```python
from build123d import *

# Parameters (mm, degrees)
F2_W = 80.009996891
F2_H = 70.8002150059
F4_T = 2.54


# Not quite as in the source:
# - the arcs of a loft's sections are written as splines that run evenly, so that the points pair up as in the source's solid
# - a shell that OpenCascade refuses in one call is made with other operations: the cavity is built on its own and cut out


with BuildPart() as f3:
    # F2 (on offset) → F3 section 0
    with BuildSketch(Plane.XY.offset(127)):
        Rectangle(F2_W, F2_H)
    # F0 (on Top) → F3 section 1
    with BuildSketch(Plane.XY):
        with BuildLine():
            add(Edge.make_bspline(
                [(26.065590987, 23.0652358186), (24.5559748328, 24.7712247593), (22.8783749167, 26.3284909791), (19.2515124469, 29.085885659), (17.3023395745, 30.2859459372), (13.2072252341, 32.2827922844), (11.0613850258, 33.0795289775), (6.6553917622, 34.2390893068), (4.3953476538, 34.6018842705), (-0.1522046827, 34.8795973285), (-2.4396004636, 34.7945085558), (-6.953951987, 34.1797019856), (-9.1807961033, 33.6499993904), (-13.4884628163, 32.1662998637), (-15.5691788974, 31.2123396195), (-19.5046195839, 28.916764877), (-21.3592468778, 27.5752071412), (-23.0652358186, 26.065590987)],
                knots=[0, 0, 0, 0, 0.125, 0.125, 0.25, 0.25, 0.375, 0.375, 0.5, 0.5, 0.625, 0.625, 0.75, 0.75, 0.875, 0.875, 1, 1, 1, 1], degree=3))
            add(Edge.make_bspline(
                [(-23.0652358186, 26.065590987), (-24.7712247593, 24.5559748328), (-26.3284909791, 22.8783749167), (-29.085885659, 19.2515124469), (-30.2859459372, 17.3023395745), (-32.2827922844, 13.2072252341), (-33.0795289775, 11.0613850258), (-34.2390893068, 6.6553917622), (-34.6018842705, 4.3953476538), (-34.8795973285, -0.1522046827), (-34.7945085558, -2.4396004636), (-34.1797019856, -6.953951987), (-33.6499993904, -9.1807961033), (-32.1662998637, -13.4884628163), (-31.2123396195, -15.5691788974), (-28.916764877, -19.5046195839), (-27.5752071412, -21.3592468778), (-26.065590987, -23.0652358186)],
                knots=[0, 0, 0, 0, 0.125, 0.125, 0.25, 0.25, 0.375, 0.375, 0.5, 0.5, 0.625, 0.625, 0.75, 0.75, 0.875, 0.875, 1, 1, 1, 1], degree=3))
            add(Edge.make_bspline(
                [(-26.065590987, -23.0652358186), (-24.5559748328, -24.7712247593), (-22.8783749167, -26.3284909791), (-19.2515124469, -29.085885659), (-17.3023395745, -30.2859459372), (-13.2072252341, -32.2827922844), (-11.0613850258, -33.0795289775), (-6.6553917622, -34.2390893068), (-4.3953476538, -34.6018842705), (0.1522046827, -34.8795973285), (2.4396004636, -34.7945085558), (6.953951987, -34.1797019856), (9.1807961033, -33.6499993904), (13.4884628163, -32.1662998637), (15.5691788974, -31.2123396195), (19.5046195839, -28.916764877), (21.3592468778, -27.5752071412), (23.0652358186, -26.065590987)],
                knots=[0, 0, 0, 0, 0.125, 0.125, 0.25, 0.25, 0.375, 0.375, 0.5, 0.5, 0.625, 0.625, 0.75, 0.75, 0.875, 0.875, 1, 1, 1, 1], degree=3))
            add(Edge.make_bspline(
                [(23.0652358186, -26.065590987), (24.7712247593, -24.5559748328), (26.3284909791, -22.8783749167), (29.085885659, -19.2515124469), (30.2859459372, -17.3023395745), (32.2827922844, -13.2072252341), (33.0795289775, -11.0613850258), (34.2390893068, -6.6553917622), (34.6018842705, -4.3953476538), (34.8795973285, 0.1522046827), (34.7945085558, 2.4396004636), (34.1797019856, 6.953951987), (33.6499993904, 9.1807961033), (32.1662998637, 13.4884628163), (31.2123396195, 15.5691788974), (28.916764877, 19.5046195839), (27.5752071412, 21.3592468778), (26.065590987, 23.0652358186)],
                knots=[0, 0, 0, 0, 0.125, 0.125, 0.25, 0.25, 0.375, 0.375, 0.5, 0.5, 0.625, 0.625, 0.75, 0.75, 0.875, 0.875, 1, 1, 1, 1], degree=3))
        make_face()
    loft(ruled=True)

    # F4: shell of thickness 2.54, made by hand


with BuildPart() as f4_core1:
    # F4_t2: copy of F3
    add(f3.part)

    # the walls: a layer under each face that stays
    f4_faces = [f4_core1.faces().sort_by_distance(p)[0] for p in [
        (37.3728696225, -1.0607857428, 63.5),
        (1.0607857428, 35.0704241512, 63.5),
        (-37.3728696225, 1.0607857428, 63.5),
        (-1.0607857428, -35.0704241512, 63.5),
        (0, 0, 0),
    ]]
    thicken(f4_faces, amount=-F4_T, mode=Mode.SUBTRACT)


with BuildPart() as f3_1:
    add(f3.part)

    # what is left inside the walls is the cavity
    f4_cavity = [f4_core1.part.solids().sort_by_distance(p)[0] for p in [
        (-0.656082, -32.618968, 85.395704),
    ]]
    add(f4_cavity, mode=Mode.SUBTRACT)


solid = f3_1.part
```
Here's how the part is built. I have some questions about the finished solid (model axes, mm). Give positions to 0.01 mm unless a question says otherwise; leave off trailing zeros. Answer as a JSON object with one key per item and string values. Group by question number.
Item 1: If we mould it in two halves opening along X, with no side actions, what happens to faces 1 (the flat face through (-1, 0, 2.54)), 2 (the flat face through (-1, 0, 0))? For each: pulls with the +X half, pulls with the -X half, needs draft (parallel to the pull), parting line crosses it, or undercut.
Item 2: For P1, Ø4, axis at x = -30.5, z = 46.5, coming from the -Y side; P2, Ø4, axis at y = 14, z = 108.5, coming from the +X side; P3, Ø1, axis at x = 3.5, y = 0.5, coming from the +Z side, each with a flat end and sliding along its axis, tell me the tip position at first contact or that it passes through.
Item 3: Please list where these lines run through material, in increasing order: probe 1 along Z at (x, y) = (-26, 10.5); probe 2 along Y at (x, z) = (21, 66.5); probe 3 along X at (y, z) = (21, 116.5).
Result set:
{
 "1": {"face 1": "undercut", "face 2": "needs draft"},
 "2": {"P1": "y = -28.87", "P2": "x = 39.18", "P3": "z = 2.54"},
 "3": {"probe 1": "0 to 2.54", "probe 2": "-33.44 to -30.86, 30.22 to 32.82", "probe 3": "-39.18 to -36.63, 36.78 to 39.33"}
}
